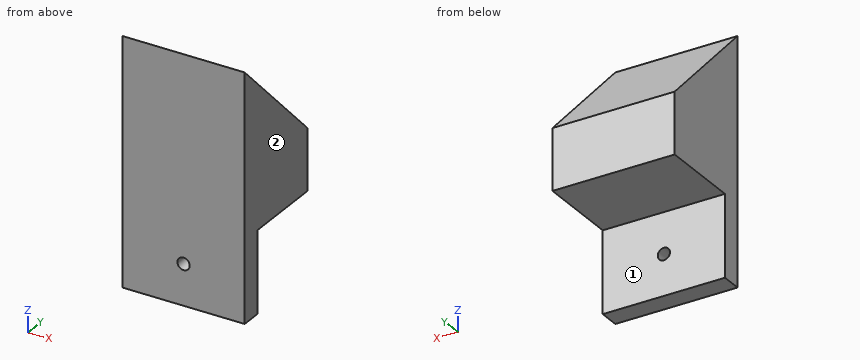
Autodesk Inventor part; units mm, degrees
ref_plane "YZ Plane" through (0, 0, 0) normal (1, 0, 0) x (0, 1, 0)
ref_plane "XZ Plane" through (0, 0, 0) normal (0, 1, 0) x (-1, 0, 0)
ref_plane "XY Plane" through (0, 0, 0) normal (0, 0, 1) x (1, 0, 0)
sketch "Skizze1" plane through (0, 0, 0) normal (1, 0, 0) x (0, 1, 0)
  line L0 (0, 0) -> (0, -40)
  line L1 (0, -40) -> (40, -40)
  line L2 (40, -40) -> (0, 0)
  dimension "d0" = 45
  dimension "d1" = 40
extrude "Extrusion1" add sketch "Skizze1" along normal blind 30
sketch "Skizze4" plane through (0, 0, -40) normal (0, 0, -1) x (-1, 0, 0)
  line L0 (-30, 0) -> (-30, 40)
  line L1 (0, 0) -> (-30, 0)
  line L2 (-30, 0) -> (-30, 5)
  line L3 (-30, 5) -> (0, 5)
  line L4 (0, 5) -> (0, 0)
  dimension "d19" = 5
extrude "Extrusion2" add sketch "Skizze4" along normal blind 20
sketch "Skizze5" plane through (0, 5, -40) normal (0, 1, 0) x (1, 0, 0)
  line L0 (30, 20) -> (0, 20) construction
  line L1 (15, 20) -> (15, 0) construction
  line L2 (0, 0) -> (30, 0) construction
  line L3 (0, 0) -> (0, 20) construction
  line L4 (30, 0) -> (0, 0) construction
  line L5 (30, 0) -> (30, 20) construction
  line L6 (0, 20) -> (30, 20) construction
  line L7 (0, 0) -> (0, 20) construction
  line L8 (0, 10) -> (30, 10) construction
  point P0 (0, -40)
  point P1 (15, 10)
hole "Bohrung2" at (15, 5, -50) direction (0, -1, 0) diameter 3 end through all
sketch "Skizze6" plane through (30, 0, 0) normal (1, 0, 0) x (0, 0, -1)
  line L0 (40, 5) -> (40, 40)
  line L1 (40, 40) -> (20, 40)
  line L2 (20, 40) -> (20, 25)
  line L3 (20, 25) -> (40, 25)
  line L4 (40, 25) -> (40, 40)
  point P0 (0, 0)
  dimension "d29" = 15
  dimension "d30" = 20
extrude "Extrusion3" cut sketch "Skizze6" against normal through all
properties part number "spiegelhalter"
Build history of the part. All positions in model axes, mm. Face numbers are marked on the shaded views. A direction names the side the tool comes from. Round coordinates to 2 decimals unless told otherwise and drop trailing zeros. Write each loop counter-clockwise with the first axis right and the second up, starting at its lowest first coordinate (ties: lowest second). Pieces come first, ordered by that corner, then holes. Notation, with made-up numbers: M 32,73.5 L 87,73.5 A19 cw 87,106.5 Z; hole C 15,57.5 d6. An arc over 180 degrees is marked long. Answer as a JSON object with one key per item and string values. Group by question number.
(1) Cut at C-C (y = 6.5). Give the cut face in (x, z), and give its area (4 significant figures).
(2) Cut at B-B (x = 15). Give the cut face in (y, z).
(3) Cut at A-A (z = -50). Give the cut face in (x, y), and give its area (3 significant figures).
(4) Flat gauge pins, fed straight in: pin 1 (3 mm diameter, centred on y = 18, z = -16, fed in from +X); pin 2 (1 mm diameter, centred on x = 11, y = 17, fed in from -Z); pin 3 (8 mm diameter, centred on x = 5.5, y = 9.5, fed in from +Z). Where does each tip first touch, or does it go through?
(5) Cut at D-D (x = 21.75). Give the cut face in (y, z), and give its area (4 significant figures).
(6) Which spindle directions (+Z, -Z, +X, -X, +Y, -Y) get a long thin tool onto all of the face, cutting with end or side? Do the marked faces 1 and 2. Say none if no direction does.
(7) Drill centre lines: L1, parallel to X at y = 1.65, z = -50; L2, parallel to Y at x = 10, z = -56.5; L3, parallel to X at y = 4.25, z = -51. Where is each one in solid material? Low to high.
Responses:
{
 "1": {"outline": "M 0,-40 L 30,-40 L 30,-6.5 L 0,-6.5 Z", "area": "1,005 mm2"},
 "2": {"outline": "M 0,-60 L 5,-60 L 5,-51.5 L 0,-51.5 Z; M 0,-48.5 L 5,-48.5 L 5,-40 L 25,-40 L 25,-25 L 0,0 Z"},
 "3": {"outline": "M 0,0 L 13.5,0 L 13.5,5 L 0,5 Z; M 16.5,0 L 30,0 L 30,5 L 16.5,5 Z", "area": "135 mm2"},
 "4": {"pin 1": "stops at x = 30", "pin 2": "stops at z = -40", "pin 3": "stops at z = -5.5"},
 "5": {"outline": "M 0,-60 L 5,-60 L 5,-40 L 25,-40 L 25,-25 L 0,0 Z", "area": "787.5 mm2"},
 "6": {"face 1": "-Z, +X, -X, +Y", "face 2": "+Z, -Z, +X, +Y, -Y"},
 "7": {"L1": "x = 0 to 13.5, 16.5 to 30", "L2": "y = 0 to 5", "L3": "x = 0 to 13.88, 16.12 to 30"}
}
